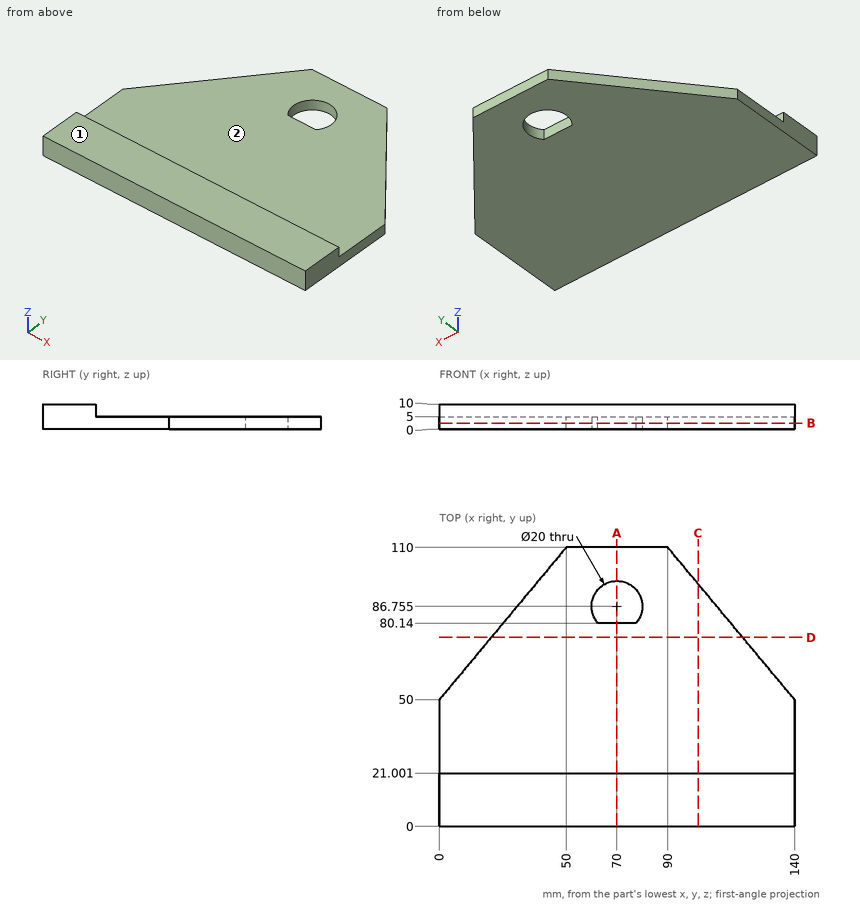
Geometry check sheet. Reference: drawing and pictorial views, mm from the part's lowest x, y, z. A direction names the side the tool comes from. Give positions to 0.01 mm unless a question says otherwise; leave off trailing zeros. Write each loop counter-clockwise with the first axis right and the second up, starting at its lowest first coordinate (ties: lowest second). Pieces come first, ordered by that corner, then holes.
Item 1: Scan lines: L1, parallel to Y at x = 70, z = 3.3 (1 decimal); L2, parallel to Y at x = 91, z = 8.5; L3, parallel to Z at x = 71.5, y = 61.5. Record each from-to range of solid material in increasing order.
Item 2: Cross-section at D-D (y = 74.5). Enter the section's corners in (x, z), and give its area (3 significant figures).
Item 3: Access from +Z, -Z, +X, -X, +Y, -Y to the whole of each face (thin tool, end or side, straight path). Record for the marked faces 1 and 2.
Item 4: Cross-section at A-A (x = 70). Enter the section's corners in (y, z) (1 decimal).
Item 5: Gauge pin test, flat ends, axial feed: pin 1 (12 mm diameter, centred on x = 32, y = 93, fed in from -Z); pin 2 (1 mm diameter, centred on x = 66, z = 8.5, fed in from +Y); pin 3 (2 mm diameter, centred on x = 38.5, y = 49, fed in from +Z). Record the tip position at first contact, or that the pin passes through.
Item 6: Cross-section at B-B (z = 2.5). Enter the section's corners in (x, y) (1 decimal).
Item 7: Cross-section at C-C (x = 102). Enter the section's corners in (y, z).
Report:
1. L1: y = 0 to 80.1, 96.8 to 110
1. L2: y = 0 to 21
1. L3: z = 0 to 5
2. outline: (20.42, 0) - (119.58, 0) - (119.58, 5) - (20.42, 5) - close
2. area: 496 mm2
3. face 1: +Z, +X, -X, +Y, -Y
3. face 2: +Z, +X, -X, +Y
4. outline: (0, 0) - (80.1, 0) - (80.1, 5) - (21, 5) - (21, 10) - (0, 10) - close; (96.8, 0) - (110, 0) - (110, 5) - (96.8, 5) - close
5. pin 1: stops at z = 0
5. pin 2: stops at y = 21
5. pin 3: stops at z = 5
6. outline: (0, 0) - (140, 0) - (140, 50) - (90, 110) - (50, 110) - (0, 50) - close; hole (62.5, 80.1) - (77.5, 80.1) arc R10 ccw (long way) to start
7. outline: (0, 0) - (95.6, 0) - (95.6, 5) - (21, 5) - (21, 10) - (0, 10) - close
